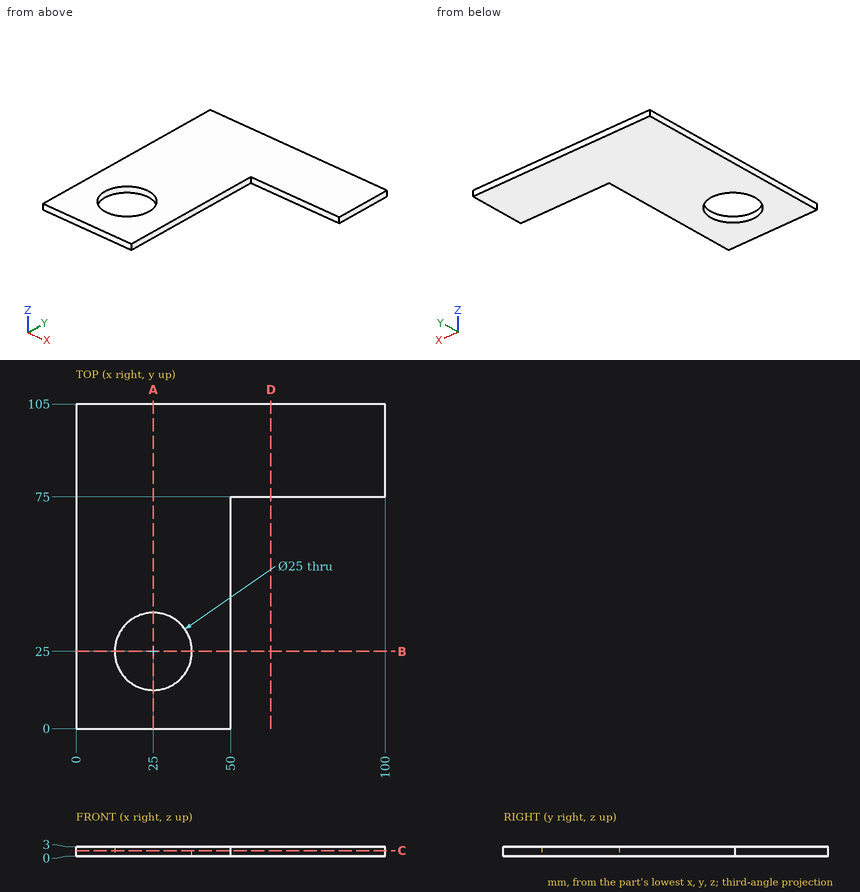
The figure shows three views and two pictorial views of one solid part (mm, origin at its lowest corner). Answer the questions. Round coordinates to 2 decimals unless told otherwise and drop trailing zeros. Write each loop counter-clockwise with the first axis right and the second up, starting at its lowest first coordinate (ties: lowest second). Pieces come first, ordered by that corner, then holes. Notation, with made-up numbers: (-36, 43.5) -> (16, 43.5) arc R15 ccw to (16, 70.5) -> close; hole circle Ø2 at (-18, 47.5). An arc over 180 degrees is marked (long way). Write each question's results on one line, items separated by ' | '.
Q1. Section B-B, the plane y = 25 is taken. Write down the section's boundary in (x, z), then the cut area to 3 significant figures.
Data:
outline: (0, 0) -> (12.5, 0) -> (12.5, 3) -> (0, 3) -> close; (37.5, 0) -> (50, 0) -> (50, 3) -> (37.5, 3) -> close | area: 75.0 mm^2
Q2. Straight lines are drawn through the part: line 1 along Y through (x, z) = (25, 1.8); line 2 along Y through (x, z) = (62, 1.3); line 3 along Y through (x, z) = (35, 2.55). For each, find the intervals that lie inside material, in ascending order. Write a range as [from, to].
Data:
line 1: [0, 12.5], [37.5, 105] | line 2: [75, 105] | line 3: [0, 17.5], [32.5, 105]
Q3. Section A-A, the plane x = 25 is taken. Write down the section's boundary in (y, z), then the cut area to 3 significant figures.
Data:
outline: (0, 0) -> (12.5, 0) -> (12.5, 3) -> (0, 3) -> close; (37.5, 0) -> (105, 0) -> (105, 3) -> (37.5, 3) -> close | area: 240 mm^2
Q4. Section D-D, the plane x = 63 is taken. Write down the section's boundary in (y, z), then the cut area to 3 significant figures.
Data:
outline: (75, 0) -> (105, 0) -> (105, 3) -> (75, 3) -> close | area: 90.0 mm^2
Q5. Section C-C, the plane z = 1.75 is taken. Write down the section's boundary in (x, y), then the cut area to 3 significant figures.
Data:
outline: (0, 0) -> (50, 0) -> (50, 75) -> (100, 75) -> (100, 105) -> (0, 105) -> close; hole circle Ø25 at (25, 25) | area: 6,260 mm^2
Q6. Flat-ended cylindrical pins translate along their axes: P1, Ø20, axis at x = 25, y = 25, coming from the +Z side; P2, Ø1.5, axis at x = 72, z = 1, coming from the -Y side. Find the tip coordinate at first contact, or state that the pin passes through.
Data:
P1: through | P2: y = 75
